Design review of the part built by this model. Coordinates are the model's own, in mm. A direction names the side the tool comes from. Round coordinates to 2 decimals unless told otherwise and drop trailing zeros. Write each loop counter-clockwise with the first axis right and the second up, starting at its lowest first coordinate (ties: lowest second). Pieces come first, ordered by that corner, then holes. Notation, with made-up numbers: (-16, 12.25) -> (4, 12.25) arc R15 ccw to (4, 38.25) -> close; hole circle Ø7 at (-13, -11.5). An arc over 180 degrees is marked (long way). Write item = value, one per line. Start each with the question number.
Item 1: Machinability: for faces 1 (the flat face through (40, 52.07, -14)), 2 (the flat face through (40, 52.578, 14)), which of the approach directions +Z, -Z, +X, -X, +Y, -Y give a long, thin tool a straight path to every point of the face, cutting with its end or side? Answer none if there is none.
Item 2: For pin 1 Ø0.5 at (y, z) = (51.5, 14) entering from +X; pin 2 Ø0.6 at (y, z) = (52.5, 15) entering from -X; pin 3 Ø0.9 at (x, y) = (39.5, 52) entering from +Z; pin 4 Ø0.5 at (x, y) = (41, 51.5) entering from +Z, all flat-tipped, find the tip position at first contact; note any pin that passes through.
Item 3: Add section C-C, the plane z = -13.5. State the section outline as (x, y) points, then the cut area to 3 significant figures.
Item 4: Add section A-A, the plane z = 8.5. State the section outline as (x, y) points.
Item 5: Add section B-B, the plane x = 18. State the section outline as (y, z) points, then the cut area to 3 significant figures.
Item 6: To check wall thickness, follow L1, parallel to Y at x = -0.5, z = 10. State the ranges of the line that lie inside material, in increasing order.
from build123d import *

# Parameters (mm, degrees)
SKETCH1_W           = 101.6
SKETCH1_H           = 40.64
BOSS_EXTRUDE1_DEPTH = 50.8
BOSS_EXTRUDE2_START = -8.89
BOSS_EXTRUDE2_DEPTH = 5.08
FILLET1_R           = 0.254


with BuildPart() as part:
    # Sketch1 → Boss-Extrude1 (new body)
    with BuildSketch(Plane(origin=(0, 0, 0), x_dir=(1, 0, 0), z_dir=(0, 1, 0))):
        Rectangle(SKETCH1_W, SKETCH1_H)
    extrude(amount=BOSS_EXTRUDE1_DEPTH)

    # Sketch3 → Boss-Extrude2 (add)
    with BuildSketch(Plane(origin=(0, 0, -20.32), x_dir=(-1, 0, 0), z_dir=(0, 0, -1)).offset(BOSS_EXTRUDE2_START)):
        Polygon((-42.418, 50.8), (-42.418, 52.578), (-38.09867671, 52.578), (-38.09867671, 52.07), (-41.91, 52.07), (-41.91, 50.8), align=None)
    boss_extrude2 = extrude(amount=BOSS_EXTRUDE2_DEPTH)

    # Mirror1: Boss-Extrude2 across plane
    add(boss_extrude2.mirror(Plane.XY))

    # Fillet1
    fillet1_edges = [part.edges().sort_by_distance(p)[0] for p in [
        (-50.8, 50.8, 0),
        (0, 50.8, 20.32),
        (41.91, 52.07, -13.97),
        (42.418, 52.578, -13.97),
        (50.8, 50.8, 0),
        (0, 0, 20.32),
        (-50.8, 0, 0),
        (42.418, 52.578, 13.97),
        (41.91, 52.07, 13.97),
        (0, 0, -20.32),
        (50.8, 0, 0),
        (0, 50.8, -20.32),
        (50.8, 25.4, 20.32),
        (-50.8, 25.4, 20.32),
        (-50.8, 25.4, -20.32),
        (50.8, 25.4, -20.32),
    ]]
    fillet(fillet1_edges, radius=FILLET1_R)


solid = part.part
Result set:
q1.face_1 = +Z, -Z, -X
q1.face_2 = +Z, -Z, +X, -X, +Y
q2.pin_1 = 42.42
q2.pin_2 = 38.1
q2.pin_3 = 16.51
q2.pin_4 = through
q3.outline = (-50.8, 0.25) arc R0.25 ccw to (-50.55, 0) -> (50.55, 0) arc R0.25 ccw to (50.8, 0.25) -> (50.8, 50.55) arc R0.25 ccw to (50.55, 50.8) -> (42.42, 50.8) -> (42.42, 52.32) arc R0.25 ccw to (42.16, 52.58) -> (38.1, 52.58) -> (38.1, 52.07) -> (41.66, 52.07) arc R0.25 cw to (41.91, 51.82) -> (41.91, 50.8) -> (-50.55, 50.8) arc R0.25 ccw to (-50.8, 50.55) -> close
q3.area = 5,160 mm²
q4.outline = (-50.8, 0.25) arc R0.25 ccw to (-50.55, 0) -> (50.55, 0) arc R0.25 ccw to (50.8, 0.25) -> (50.8, 50.55) arc R0.25 ccw to (50.55, 50.8) -> (-50.55, 50.8) arc R0.25 ccw to (-50.8, 50.55) -> close
q5.outline = (0, -20.07) arc R0.25 ccw to (0.25, -20.32) -> (50.55, -20.32) arc R0.25 ccw to (50.8, -20.07) -> (50.8, 20.07) arc R0.25 ccw to (50.55, 20.32) -> (0.25, 20.32) arc R0.25 ccw to (0, 20.07) -> close
q5.area = 2,060 mm²
q6.L1 = 0 to 50.8
